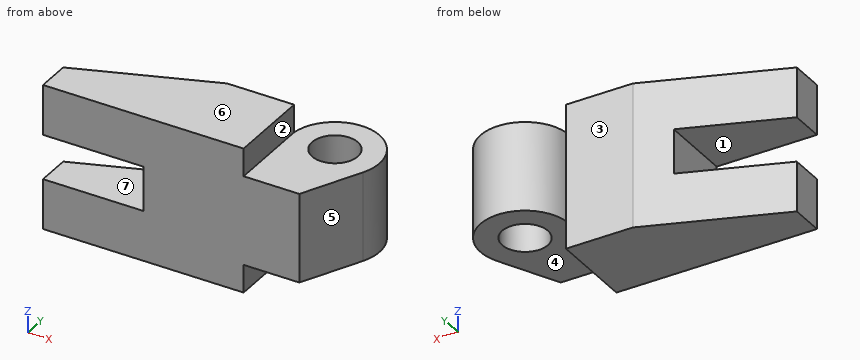
from build123d import *

# Parameters (mm, degrees)
BOSS_EXTRUDE2_DEPTH      = 13
BOSS_EXTRUDE2_DEPTH_BACK = 13
SKETCH3_W                = 18
SKETCH3_H                = 8
CUT_EXTRUDE2_DEPTH       = 27.795522014
BOSS_EXTRUDE3_DEPTH      = 8
BOSS_EXTRUDE3_DEPTH_BACK = 8
SKETCH5_R                = 4.1
CUT_EXTRUDE3_DEPTH       = 43.46159682


with BuildPart() as part:
    # Sketch1 → Boss-Extrude2 (new, two sides: drawn at the far end of the back side and taken through both)
    with BuildSketch(Plane.XY.offset(-BOSS_EXTRUDE2_DEPTH_BACK)):
        Polygon((-18, -1.5), (6, 7.5), (18, 7.5), (18, -7.5), (-18, -7.5), align=None)
    extrude(amount=BOSS_EXTRUDE2_DEPTH + BOSS_EXTRUDE2_DEPTH_BACK)

    # Sketch3 → Cut-Extrude2 (cut, through all)
    with BuildSketch(Plane.XZ.offset(7.5)):
        with Locations((-9, 0)):
            Rectangle(SKETCH3_W, SKETCH3_H)
    extrude(amount=-CUT_EXTRUDE2_DEPTH, mode=Mode.SUBTRACT)

    # Sketch4 → Boss-Extrude3 (add, two sides: drawn at the far end of the back side and taken through both)
    with BuildSketch(Plane.XY.offset(-BOSS_EXTRUDE3_DEPTH_BACK)):
        with BuildLine():
            Line((18, 7.5), (18, -7.5))
            Line((18, -7.5), (28, -7.5))
            Line((28, -7.5), (33.12495505, 2.987600158))
            ThreePointArc((33.12495505, 2.987600158), (28.224369024, 14.166101001), (18, 7.5))
        make_face()
    extrude(amount=BOSS_EXTRUDE3_DEPTH + BOSS_EXTRUDE3_DEPTH_BACK)

    # Sketch5 → Cut-Extrude3 (cut, through all)
    with BuildSketch(Plane.XY.offset(8)):
        with Locations((25.937253933, 6.5)):
            Circle(SKETCH5_R)
    extrude(amount=-CUT_EXTRUDE3_DEPTH, mode=Mode.SUBTRACT)


solid = part.part
Read the model definition and answer for the solid it produces. Units are mm, in the model's axes. Face numbers are marked on the shaded views. A direction names the side the tool comes from. Round coordinates to 2 decimals unless told otherwise and drop trailing zeros. Order: outer loops, then holes, each group sorted by start corner. A loop starts at its lowest first (then second) coordinate and runs counter-clockwise, first axis right, second up. Notation, with made-up numbers: (61.25, 87.25) - (88.25, 87.25) arc R22 ccw to (88.25, 121.25) - close; hole circle Ø10 at (78.5, -36). An arc over 180 degrees is marked (long way). Use one line per item in the form item = value. Start each with the question number.
(1) The part is cut by section A-A (x = -2). Give the vertices of the cut face in (y, z), then the cut area to 3 significant figures.
(2) For the marked faces 1, 2, 3 and 4, determine the directions among +Z, -Z, +X, -X, +Y, -Y from which every point of the face is accessible in a straight line to the end or side of a thin tool.
(3) Find the intervals of material crossed by line 1 along Z through (x, y) = (-5.5, 2.75); line 2 along Z through (x, y) = (19, -4.5); line 3 along X through (y, z) = (-3, -11), in increasing order. Write a range as from..to.
(4) The part is cut by section C-C (z = 8.75). Give the vertices of the cut face in (x, y), then the cut area to 3 significant figures.
(5) The part is cut by section B-B (y = 4.25). Give the vertices of the cut face in (x, z), then the cut area to 3 significant figures.
(6) The part is cut by section D-D (y = -0.25). Give the vertices of the cut face in (x, z), then the cut area to 3 significant figures.
(7) Flat-ended cylindrical pins translate along their axes: pin 1 Ø8 at (x, z) = (-7.5, 3) entering from +Y; pin 2 Ø12.5 at (x, y) = (26, 4.5) entering from +Z; pin 3 Ø4 at (y, z) = (0, -0.5) entering from -X. Find the tip coordinate at first contact, or state that the pin passes through.
(8) Determine the mould class of the marked faces 5, 6 and 7 for opening direction Z: +Z half, -Z half, draft (parallel to the pull), parting line (faces both ways), or undercut.
Checked values:
q1.outline = (-7.5, -13) - (4.5, -13) - (4.5, -4) - (-7.5, -4) - close; (-7.5, 4) - (4.5, 4) - (4.5, 13) - (-7.5, 13) - close
q1.area = 216 mm^2
q2.face_1 = -X, +Y, -Y
q2.face_2 = +Z, +X, +Y, -Y
q2.face_3 = +Z, -Z, -X, +Y
q2.face_4 = -Z, +X, +Y, -Y
q3.line_1 = -13..-4, 4..13
q3.line_2 = -8..8
q3.line_3 = -18..18
q4.outline = (-18, -7.5) - (18, -7.5) - (18, 7.5) - (6, 7.5) - (-18, -1.5) - close
q4.area = 432 mm^2
q5.outline = (-2.67, -13) - (18, -13) - (18, -8) - (22.51, -8) - (22.51, 8) - (18, 8) - (18, 13) - (-2.67, 13) - (-2.67, 4) - (0, 4) - (0, -4) - (-2.67, -4) - close; (29.36, -8) - (33.61, -8) - (33.61, 8) - (29.36, 8) - close
q5.area = 656 mm^2
q6.outline = (-14.67, -13) - (18, -13) - (18, -8) - (31.54, -8) - (31.54, 8) - (18, 8) - (18, 13) - (-14.67, 13) - (-14.67, 4) - (0, 4) - (0, -4) - (-14.67, -4) - close
q6.area = 949 mm^2
q7.pin_1 = 3.89
q7.pin_2 = 8
q7.pin_3 = 0
q8.face_5 = draft
q8.face_6 = +Z half
q8.face_7 = undercut
